For this review, use the dimensioned drawing (mm, ordinates from the lowest corner) and the shaded views. Give positions to 0.01 mm unless a question says otherwise; leave off trailing zeros. Loops run counter-clockwise (first coordinate to the right, second up) from the corner with the lowest first, then second, coordinate; pieces in that order, holes last. Notation, with made-up numbers: (45, 83) -> (61, 83) arc R30 cw to (61, 109) -> close; hole circle Ø10 at (-39.5, -8). An arc over 180 degrees is marked (long way). Write each question's results on one line, items separated by ' | '. Start each with the question number.
Q1. We need section A-A (x = 30.5). Write out the cut boundary in (y, z), plus the area to 3 significant figures.
Q2. Insertion check: pin 1 Ø7.5 at (x, z) = (9, 9.5) entering from -Y; pin 2 Ø7.5 at (x, z) = (333, 11) entering from +Y; pin 3 Ø7.5 at (y, z) = (17, 5) entering from +X. Each pin has a flat end and moves straight along its axis. Give the tip position at first contact, or say it passes through.
Q3. We need section B-B (y = 306). Write out the cut boundary in (x, z).
Q4. Wall thickness on L1, parallel to Y at x = 324, z = 9.5; L2, parallel to X at y = 374, z = 9.75; L3, parallel to X at y = 314.5, z = 12: over which ranges is each line inside the solid? List them lowest first. Write a range as [from, to].
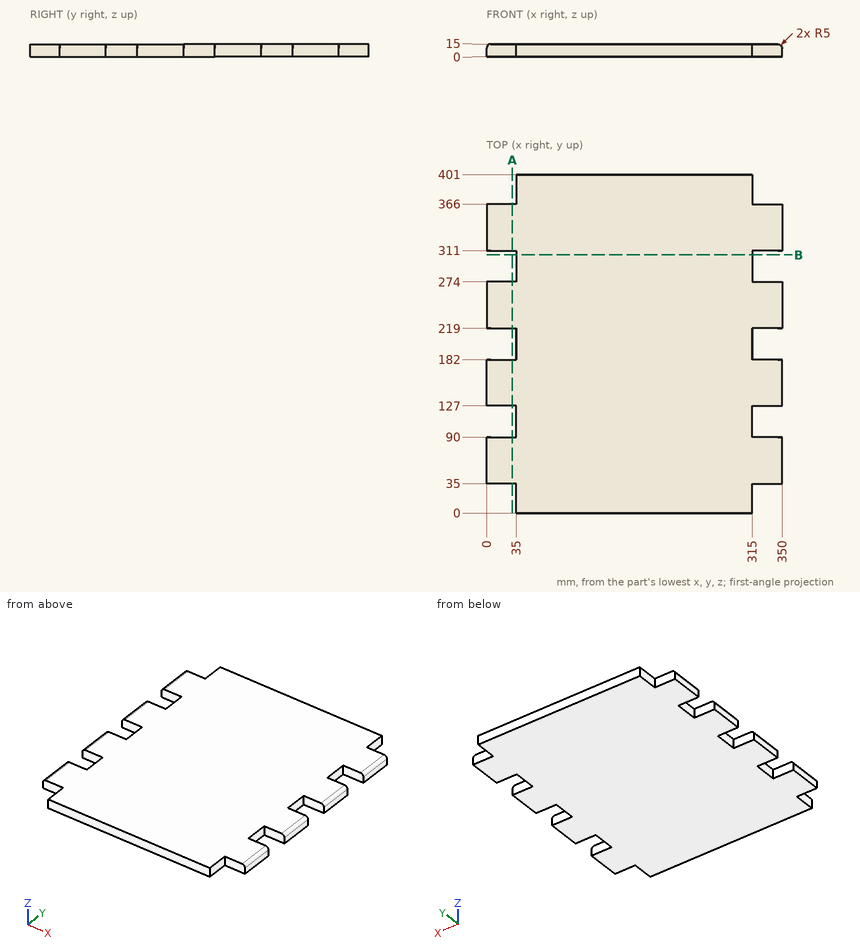
Output:
1) outline: (35, 0) -> (90, 0) -> (90, 15) -> (35, 15) -> close; (127, 0) -> (182, 0) -> (182, 15) -> (127, 15) -> close; (219, 0) -> (274, 0) -> (274, 15) -> (219, 15) -> close; (311, 0) -> (366, 0) -> (366, 15) -> (311, 15) -> close | area: 3,300 mm2
2) pin 1: y = 35 | pin 2: y = 366 | pin 3: x = 315
3) outline: (35, 0) -> (315, 0) -> (315, 15) -> (35, 15) -> close
4) L1: [35, 90], [127, 182], [219, 274], [311, 366] | L2: [35, 315] | L3: [0.42, 349.58]
